```python
from build123d import *

# Parameters (mm, degrees)
SKETCH1_W          = 5
SKETCH1_H          = 6.6
CUT_EXTRUDE1_DEPTH = 6.6
CUT_EXTRUDE2_DEPTH = 6.6
CUT_EXTRUDE3_DEPTH = 6.6
CHAMFER1_SIZE      = 0.5


with BuildPart() as part:
    # Sketch1 → Revolve-Thin1 (revolve)
    with BuildSketch(Plane(origin=(0, 0, 0), x_dir=(1, 0, 0), z_dir=(0, 1, 0))):
        with Locations((-2.5, 20.8)):
            Rectangle(SKETCH1_W, SKETCH1_H)
    revolve(axis=Axis((0, 0, 0), (0, 0, -1)))

    # Sketch3 → Revolve-Thin2 (revolve)
    with BuildSketch(Plane(origin=(0, 0, 0), x_dir=(1, 0, 0), z_dir=(0, 1, 0))):
        Polygon((-27.192355447, 70.553826822), (0, 20.8), (4.387478051, 23.197923342), (-22.804877396, 72.951750164), align=None)
    revolve(axis=Axis((-27.192355447, 0, -70.553826822), (0.479584668, 0, 0.87749561)))

    # Sketch4 → Revolve-Thin3 (revolve)
    with BuildSketch(Plane(origin=(0, 0, 0), x_dir=(1, 0, 0), z_dir=(0, 1, 0))):
        Polygon((0, 20.8), (27.192355447, 70.553826822), (22.804877396, 72.951750164), (-4.387478051, 23.197923342), align=None)
    revolve(axis=Axis((0, 0, -20.8), (0.479584668, 0, -0.87749561)))

    # Sketch5 → Cut-Extrude1 (cut)
    with BuildSketch(Plane(origin=(-35.945691024, 0, -65.769796576), x_dir=(-0.87749561, 0, 0.479584668), z_dir=(-0.479584668, 0, -0.87749561))):
        Polygon((-7.021637489, 1.286202481), (-9.612383318, 3.201100925), (-12.566106931, 1.914898444), (-12.929084714, -1.286202481), (-10.338338885, -3.201100925), (-7.384615273, -1.914898444), align=None)
    extrude(amount=-CUT_EXTRUDE1_DEPTH, mode=Mode.SUBTRACT)

    # Sketch6 → Cut-Extrude2 (cut)
    with BuildSketch(Plane.XY.offset(-17.5)):
        Polygon((1.610807251, 2.79), (-1.610807251, 2.79), (-3.221614502, 0), (-1.610807251, -2.79), (1.610807251, -2.79), (3.221614502, 0), align=None)
    extrude(amount=-CUT_EXTRUDE2_DEPTH, mode=Mode.SUBTRACT)

    # Sketch7 → Cut-Extrude3 (cut)
    with BuildSketch(Plane(origin=(35.945691024, 0, -65.769796576), x_dir=(-0.87749561, 0, -0.479584668), z_dir=(0.479584668, 0, -0.87749561))):
        Polygon((9.612383318, 3.201100925), (7.021637489, 1.286202481), (7.384615273, -1.914898444), (10.338338885, -3.201100925), (12.929084714, -1.286202481), (12.566106931, 1.914898444), align=None)
    extrude(amount=-CUT_EXTRUDE3_DEPTH, mode=Mode.SUBTRACT)

    # Chamfer1
    chamfer1_edges = [part.edges().sort_by_distance(p)[0] for p in [
        (-29.624979245, -0.314347981, -69.224305553),
        (-28.647550905, 2.243651703, -69.758507252),
        (-26.214927107, 2.557999684, -71.088028522),
        (-24.75973165, 0.314347981, -71.883348091),
        (-25.73715999, -2.243651703, -71.349146391),
        (-28.169783788, -2.557999684, -70.019625122),
        (2.416210877, 1.395, -17.5),
        (0, 2.79, -17.5),
        (-2.416210877, 1.395, -17.5),
        (-2.416210877, -1.395, -17.5),
        (0, -2.79, -17.5),
        (2.416210877, -1.395, -17.5),
        (26.214927107, 2.557999684, -71.088028522),
        (28.647550905, 2.243651703, -69.758507252),
        (29.624979245, -0.314347981, -69.224305553),
        (28.169783788, -2.557999684, -70.019625122),
        (25.73715999, -2.243651703, -71.349146391),
        (24.75973165, 0.314347981, -71.883348091),
    ]]
    chamfer(chamfer1_edges, length=CHAMFER1_SIZE)


solid = part.part
```
Verification items for the finished model (mm, model axes). A direction names the side the tool comes from. Give positions to 0.01 mm unless a question says otherwise; leave off trailing zeros. Use a Markdown table: item, result.
1) Material ranges on probe 1 along X at (y, z) = (0.75, -64); probe 2 along X at (y, z) = (1.5, -65); probe 3 along X at (y, z) = (3.5, -60.5), recorded low to high.
Results:
| item | result |
|---|---|
| probe 1 | -29.24 to -26.91, -25.42 to -17.98, 17.98 to 25.42, 26.91 to 29.24 |
| probe 2 | -29.59 to -27.19, -23.59 to -18.72, 18.72 to 23.59, 27.19 to 29.59 |
| probe 3 | -25.77 to -17.63, 17.63 to 25.77 |
2) Mould release check, pull along Y, two halves, no side actions. Record for faces 5 (the flat face through (2.405, -1.415, -21.007)), 6 (the flat face through (-28.229, -3.263, -69.987)), 7 (the cylindrical face through (-4.77, 1.5, -18.81)), 8 (the flat face through (-2.427, -1.375, -21.007)): pulls with the +Y half, pulls with the -Y half, needs draft (parallel to the pull), parting line crosses it, or undercut.
Results:
| item | result |
|---|---|
| face 5 | undercut |
| face 6 | needs draft |
| face 7 | parting line crosses it |
| face 8 | undercut |
3) Tool access check on faces 1 (the flat face through (-23.991, 0.045, -64.782)), 2 (the flat face through (25.986, 2.773, -70.924)), 3 (the flat face through (0, 2.79, -21)), 4 (the flat face through (-25.47, -2.43, -71.21)). Record the directions out of +Z, -Z, +X, -X, +Y, -Y that give a thin tool (end or side, any length) a straight path to the whole face; none if there is none.
Results:
| item | result |
|---|---|
| face 1 | none |
| face 2 | -Z, +X |
| face 3 | +Z |
| face 4 | -Z, -X |
4) Depth check by flat-ended pin: pin 1 Ø2.5 at (x, z) = (-0.5, -20) entering from +Y; pin 2 Ø2 at (x, y) = (17, -1.5) entering from -Z; pin 3 Ø1.7 at (x, y) = (-1, -0.5) entering from +Z; pin 4 Ø2 at (y, z) = (0.5, -26) entering from -X. Enter the tip coordinate at first touch or a pass-through.
Results:
| item | result |
|---|---|
| pin 1 | y = 5 |
| pin 2 | z = -63.77 |
| pin 3 | z = -24.1 |
| pin 4 | x = -9.07 |
